CAD build for the part. Positions are in the model's coordinates, mm. Coordinates: 2 decimals unless noted, no trailing zeros. Loops run counter-clockwise (first coordinate to the right, second up) from the corner with the lowest first, then second, coordinate; pieces in that order, holes last. Notation, with made-up numbers: (76.25, -23.75) -> (82.25, -23.75) arc R30 ccw to (82.25, 11.25) -> close; hole circle Ø10 at (75.5, -8). An arc over 180 degrees is marked (long way). Return JSON: item names as keys, results as strings. Group by question number.
(1) Flat gauge pins, fed straight in: pin 1 Ø0.9 at (y, z) = (2, 0) entering from +X; pin 2 Ø1.5 at (y, z) = (1, 0) entering from -X. Where does each tip first touch, or does it go through?
(2) Saw through at A-A on x = 17. Write the cut outline in (y, z).
(3) Saw through at B-B on z = -22. Write the cut outline in (x, y).
(4) Probe L1, parallel to X at y = -1.15, z = 22; L2, parallel to Y at x = 18, z = 1; L3, parallel to Z at x = 6, y = 0.55. List the from-to ranges inside material, lowest first.
(5) Saw through at D-D on x = 5. Write the cut outline in (y, z).
(6) Saw through at C-C on z = 17. Write the cut outline in (x, y).
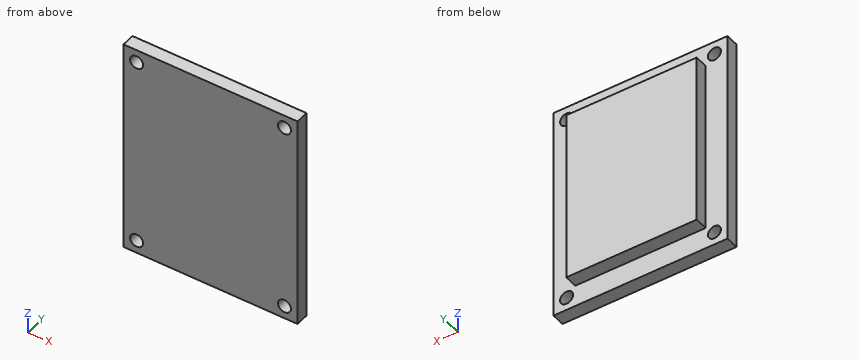
```python
from build123d import *

# Parameters (mm, degrees)
SKETCH1_W           = 30
SKETCH1_H           = 40
BOSS_EXTRUDE1_DEPTH = 3
SKETCH2_W           = 40
SKETCH2_H           = 50
SKETCH2_R           = 1.5
BOSS_EXTRUDE2_DEPTH = 3


with BuildPart() as part:
    # Sketch1 → Boss-Extrude1 (new body)
    with BuildSketch(Plane(origin=(0, 0, 0), x_dir=(1, 0, 0), z_dir=(0, 1, 0))):
        Rectangle(SKETCH1_W, SKETCH1_H)
    extrude(amount=BOSS_EXTRUDE1_DEPTH)

    # Sketch2 → Boss-Extrude2 (add)
    with BuildSketch(Plane(origin=(0, 0, 0), x_dir=(1, 0, 0), z_dir=(0, 1, 0))):
        Rectangle(SKETCH2_W, SKETCH2_H)
        with Locations(Location((-17, 21.998038487, 0), (0, 0, 270))):
            Circle(SKETCH2_R, mode=Mode.SUBTRACT)
        with Locations(Location((17, 22, 0), (0, 0, 270))):
            Circle(SKETCH2_R, mode=Mode.SUBTRACT)
        with Locations(Location((17, -22, 0), (0, 0, 270))):
            Circle(SKETCH2_R, mode=Mode.SUBTRACT)
        with Locations(Location((-17, -22, 0), (0, 0, 270))):
            Circle(SKETCH2_R, mode=Mode.SUBTRACT)
    extrude(amount=-BOSS_EXTRUDE2_DEPTH)


solid = part.part
```
Geometry results:
{
 "1": {"pin 1": "x = 15", "pin 2": "x = -15"},
 "2": {"outline": "(-3, -25) -> (0, -25) -> (0, -23.5) -> (-3, -23.5) -> close; (-3, -20.5) -> (0, -20.5) -> (0, 20.5) -> (-3, 20.5) -> close; (-3, 23.5) -> (0, 23.5) -> (0, 25) -> (-3, 25) -> close"},
 "3": {"outline": "(-20, -3) -> (-18.5, -3) -> (-18.5, 0) -> (-20, 0) -> close; (-15.5, -3) -> (15.5, -3) -> (15.5, 0) -> (-15.5, 0) -> close; (18.5, -3) -> (20, -3) -> (20, 0) -> (18.5, 0) -> close"},
 "4": {"L1": "-20 to -18.5, -15.5 to 15.5, 18.5 to 20", "L2": "-3 to 0", "L3": "-20 to 20"},
 "5": {"outline": "(-3, -25) -> (0, -25) -> (0, -20) -> (3, -20) -> (3, 20) -> (0, 20) -> (0, 25) -> (-3, 25) -> close"},
 "6": {"outline": "(-20, -3) -> (20, -3) -> (20, 0) -> (15, 0) -> (15, 3) -> (-15, 3) -> (-15, 0) -> (-20, 0) -> close"}
}
